```python
from build123d import *

# Parameters (mm, degrees)
BOSS_EXTRUDE2_DEPTH = 24
SKETCH2_R           = 4
CUT_EXTRUDE1_DEPTH  = 523.057621341


with BuildPart() as part:
    # Sketch1 → Boss-Extrude2 (new body)
    with BuildSketch(Plane.XY):
        with BuildLine():
            Line((20, 29.6), (500, 29.6))
            ThreePointArc((500, 29.6), (507.071067812, 26.671067812), (510, 19.6))
            Line((510, 19.6), (510, 0))
            Line((510, 0), (520, 0))
            Line((520, 0), (520, 19.6))
            ThreePointArc((520, 19.6), (514.142135624, 33.742135624), (500, 39.6))
            Line((500, 39.6), (20, 39.6))
            ThreePointArc((20, 39.6), (5.857864376, 33.742135624), (0, 19.6))
            Line((0, 19.6), (0, 0))
            Line((0, 0), (10, 0))
            Line((10, 0), (10, 19.6))
            ThreePointArc((10, 19.6), (12.928932188, 26.671067812), (20, 29.6))
        make_face()
    extrude(amount=BOSS_EXTRUDE2_DEPTH)

    # Sketch2 → Cut-Extrude1 (cut, through all)
    with BuildSketch(Plane.ZY):
        with Locations((12, 11)):
            Circle(SKETCH2_R)
    extrude(amount=-CUT_EXTRUDE1_DEPTH, mode=Mode.SUBTRACT)


solid = part.part
```
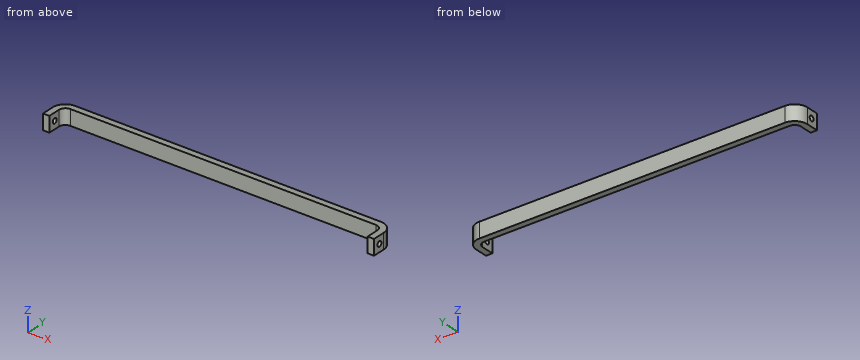
Geometry check sheet. Reference: the model listing, model coordinates, mm. Give positions to 0.01 mm unless a question says otherwise; leave off trailing zeros. Write each loop counter-clockwise with the first axis right and the second up, starting at its lowest first coordinate (ties: lowest second). Pieces come first, ordered by that corner, then holes. Notation, with made-up numbers: (-39, -19) -> (9, -19) arc R17 cw to (9, -1) -> close; hole circle Ø6 at (26, -21). An arc over 180 degrees is marked (long way). Use one line per item in the form item = value.
Item 1: Sectioned sample at A-A on z = 12. Enter the section's corners in (x, y), plus the area to 3 significant figures.
Results list:
outline = (0, 0) -> (10, 0) -> (10, 7) -> (0, 7) -> close; (0, 15) -> (10, 15) -> (10, 19.6) arc R10 cw to (20, 29.6) -> (500, 29.6) arc R10 cw to (510, 19.6) -> (510, 15) -> (520, 15) -> (520, 19.6) arc R20 ccw to (500, 39.6) -> (20, 39.6) arc R20 ccw to (0, 19.6) -> close; (510, 0) -> (520, 0) -> (520, 7) -> (510, 7) -> close
area = 5,500 mm2
Item 2: Depth check by flat-ended pin: pin 1 Ø5 at (x, z) = (86.5, 10) entering from -Y. Enter the tip coordinate at first touch or a pass-through.
Results list:
pin_1 = 29.6
Item 3: Sectioned sample at B-B on x = 257. Enter the section's corners in (y, z).
Results list:
outline = (29.6, 0) -> (39.6, 0) -> (39.6, 24) -> (29.6, 24) -> close
Item 4: Scan lines: line 1 (X direction, y = 21, z = 2.25); line 2 (X direction, y = 6, z = 9); line 3 (Y direction, x = 307.5, z = 11.75). Record each from-to range of solid material in increasing order.
Results list:
line_1 = 0.05 to 10.1, 509.9 to 519.95
line_2 = 0 to 10, 510 to 520
line_3 = 29.6 to 39.6
